For this review, use the dimensioned drawing (mm, ordinates from the lowest corner) and the shaded views. A direction names the side the tool comes from. Round coordinates to 2 decimals unless told otherwise and drop trailing zeros. Loops run counter-clockwise (first coordinate to the right, second up) from the corner with the lowest first, then second, coordinate; pieces in that order, holes last. Notation, with made-up numbers: (16.25, 30) -> (22.25, 30) arc R16 cw to (22.25, 50) -> close; hole circle Ø7 at (87, 35). An arc over 180 degrees is marked (long way). Answer as CSV lines item,"result". Start each with the question number.
(1) Machinability: for the marked faces 1, 2 and 3, which of the approach directions +Z, -Z, +X, -X, +Y, -Y give a long, thin tool a straight path to every point of the face, cutting with its end or side? Answer none if there is none.
(2) Take a section at A-A, the plane y = 19. Write out the cut boundary in (x, z).
(3) Take a section at C-C, the plane z = 17. Write out the cut boundary in (x, y).
(4) Take a section at D-D, the plane x = 23. Write out the cut boundary in (y, z).
(5) To check wall thickness, follow line 1 (X direction, y = 35.5, z = 19.75); line 2 (Y direction, x = 33, z = 18.75); line 3 (Z direction, x = 3, y = 28). State the ranges of each line that lie inside material, in increasing order. Write a range as from..to.
(6) For P1, Ø4.5, axis at y = 44.5, z = 17.5, coming from the -X side; P2, Ø2.5, axis at y = 12.5, z = 11.5, coming from the -X side; P3, Ø22, axis at x = 37.5, y = 8, coming from the +Z side, all flat-tipped, find the tip position at first contact; note any pin that passes through.
(7) Take a section at B-B, the plane x = 29. Write out the cut boundary in (y, z), and give its area (3 significant figures).
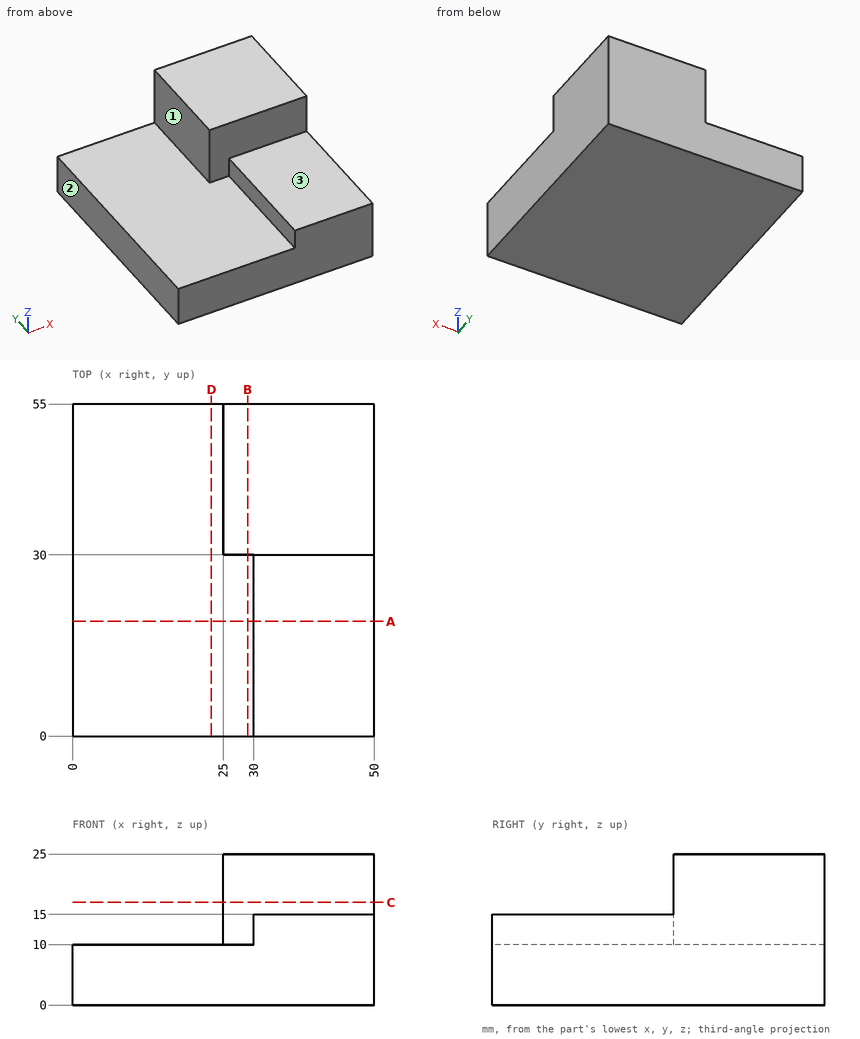
The answers:
1,face 1,"+Z, -X, +Y, -Y"
1,face 2,"+Z, -Z, -X, +Y, -Y"
1,face 3,"+Z, +X, -X, -Y"
2,outline,"(0, 0) -> (50, 0) -> (50, 15) -> (30, 15) -> (30, 10) -> (0, 10) -> close"
3,outline,"(25, 30) -> (50, 30) -> (50, 55) -> (25, 55) -> close"
4,outline,"(0, 0) -> (55, 0) -> (55, 10) -> (0, 10) -> close"
5,line 1,"25..50"
5,line 2,"30..55"
5,line 3,"0..10"
6,P1,"x = 25"
6,P2,"x = 30"
6,P3,"z = 15"
7,outline,"(0, 0) -> (55, 0) -> (55, 25) -> (30, 25) -> (30, 10) -> (0, 10) -> close"
7,area,"925 mm²"
